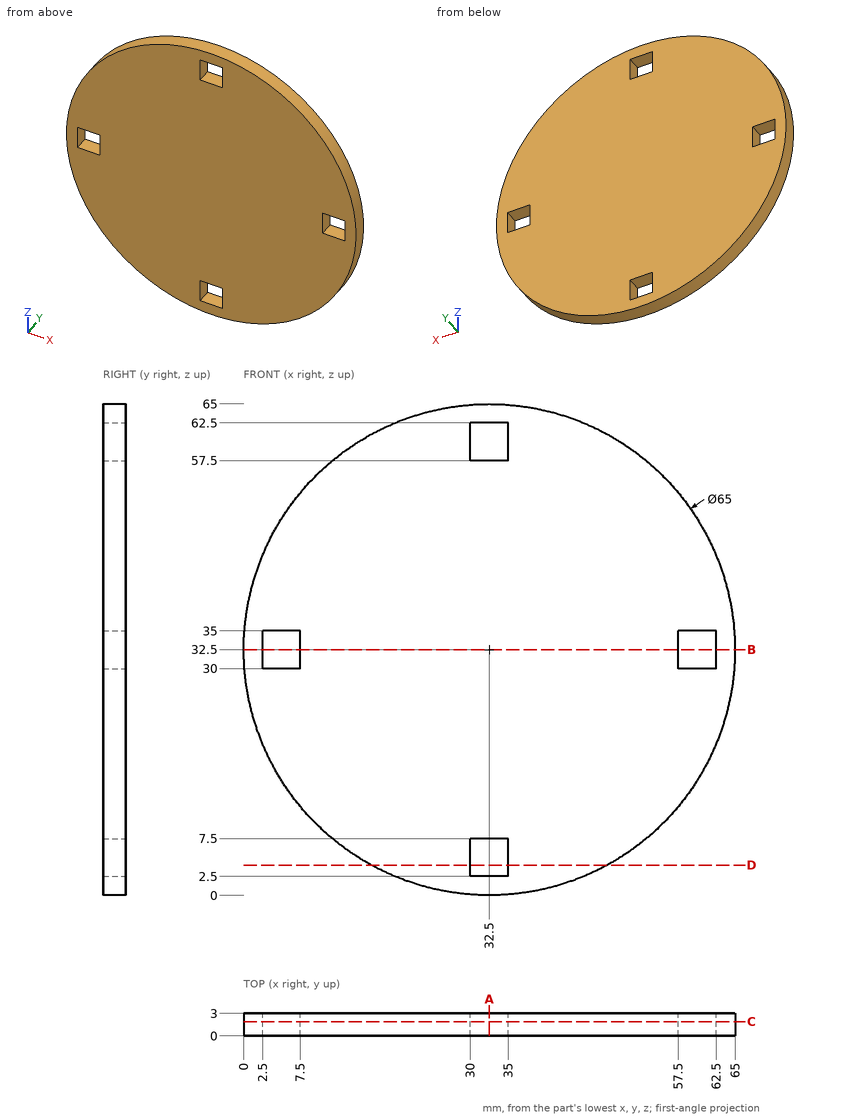
Geometry: see drawing. Coordinates: mm, zero at the bounding-box minimum. Round coordinates to 2 decimals unless told otherwise and drop trailing zeros. Loops run counter-clockwise (first coordinate to the right, second up) from the corner with the lowest first, then second, coordinate; pieces in that order, holes last. Notation, with made-up numbers: (-22.75, 53) - (11.25, 53) arc R21 cw to (11.25, 59) - close; hole circle Ø3 at (-0.75, 30). An arc over 180 degrees is marked (long way). Use CSV: the item, a comma, the result in double quotes.
Q1. Section query B-B, the plane z = 32.5. Output: boundary loops of the cut face in (x, y).
Reported:
outline,"(0, 0) - (2.5, 0) - (2.5, 3) - (0, 3) - close; (7.5, 0) - (57.5, 0) - (57.5, 3) - (7.5, 3) - close; (62.5, 0) - (65, 0) - (65, 3) - (62.5, 3) - close"
Q2. Pin query (flat end, axial travel): pin 1 Ø1.5 at (x, y) = (60, 1.5) entering from -Z; pin 2 Ø1 at (x, y) = (19.5, 2) entering from -Z; pin 3 Ø0.9 at (y, z) = (2, 33.5) entering from +X; pin 4 Ø0.9 at (x, y) = (32, 1.5) entering from +Z. Return the tip coordinate at first contact, or that it passes through.
Reported:
pin 1,"z = 14.04"
pin 2,"z = 2.5"
pin 3,"x = 65"
pin 4,"z = 65"
Q3. Section query C-C, the plane y = 1.9. Output: boundary loops of the cut face in (x, z), then the cut area to 3 significant figures.
Reported:
outline,"circle Ø65 at (32.5, 32.5); hole (2.5, 30) - (7.5, 30) - (7.5, 35) - (2.5, 35) - close; hole (30, 2.5) - (35, 2.5) - (35, 7.5) - (30, 7.5) - close; hole (30, 57.5) - (35, 57.5) - (35, 62.5) - (30, 62.5) - close; hole (57.5, 30) - (62.5, 30) - (62.5, 35) - (57.5, 35) - close"
area,"3,220 mm^2"
Q4. Section query D-D, the plane z = 4. Output: boundary loops of the cut face in (x, y).
Reported:
outline,"(16.88, 0) - (30, 0) - (30, 3) - (16.88, 3) - close; (35, 0) - (48.12, 0) - (48.12, 3) - (35, 3) - close"
Q5. Ray query, line 1 along Z through (x, y) = (33.5, 2.55); line 2 along X through (y, z) = (1.95, 3.5); line 3 along X through (y, z) = (1.55, 60.5). Return the intervals inside material, ascending.
Reported:
line 1,"0.02 to 2.5, 7.5 to 57.5, 62.5 to 64.98"
line 2,"17.83 to 30, 35 to 47.17"
line 3,"16 to 30, 35 to 49"
Q6. Section query A-A, the plane x = 32.5. Output: boundary loops of the cut face in (y, z).
Reported:
outline,"(0, 0) - (3, 0) - (3, 2.5) - (0, 2.5) - close; (0, 7.5) - (3, 7.5) - (3, 57.5) - (0, 57.5) - close; (0, 62.5) - (3, 62.5) - (3, 65) - (0, 65) - close"
